Here's how the part is built. I have some questions about the finished solid (model axes, mm). A direction names the side the tool comes from. Round coordinates to 2 decimals unless told otherwise and drop trailing zeros. Loops run counter-clockwise (first coordinate to the right, second up) from the corner with the lowest first, then second, coordinate; pieces in that order, holes last. Notation, with made-up numbers: M 48.25,-24.5 L 77.25,-24.5 A11 ccw 77.25,-14.5 Z; hole C 77,25 d10. An arc over 180 degrees is marked long. Use a Markdown table: item, result.
```python
from build123d import *

# Parameters (mm, degrees)
BOSS_EXTRUDE1_DEPTH = 215.9


with BuildPart() as part:
    # Sketch1 → Boss-Extrude1 (new body)
    with BuildSketch(Plane(origin=(0, 0, 0), x_dir=(0, 0, -1), z_dir=(1, 0, 0))):
        with BuildLine():
            Line((0, 0), (30, 0))
            Line((30, 0), (30, 5))
            Line((30, 5), (27.221875, 7.778125))
            Line((27.221875, 7.778125), (27.221875, 14.278125))
            ThreePointArc((27.221875, 14.278125), (28.035568974, 16.242556026), (30, 17.05625))
            Line((30, 17.05625), (30, 20.221875))
            ThreePointArc((30, 20.221875), (28.035568974, 21.035568974), (27.221875, 23))
            Line((27.221875, 23), (2.778125, 23))
            ThreePointArc((2.778125, 23), (1.964431026, 21.035568974), (0, 20.221875))
            Line((0, 20.221875), (0, 17.05625))
            ThreePointArc((0, 17.05625), (1.964431026, 16.242556026), (2.778125, 14.278125))
            Line((2.778125, 14.278125), (2.778125, 7.778125))
            Line((2.778125, 7.778125), (0, 5))
            Line((0, 5), (0, 0))
        make_face()
    extrude(amount=BOSS_EXTRUDE1_DEPTH)


solid = part.part
```
Q1. Will these pins go through, and if not, where does the flat tip stop? P1, Ø1.9, axis at x = 133, y = 10, coming from the -Z side; P2, Ø3, axis at x = 63, y = 8.5, coming from the +Z side; P3, Ø3, axis at x = 93, y = 11, coming from the +Z side.
Return value:
| item | result |
|---|---|
| P1 | stops at z = -27.22 |
| P2 | stops at z = -2 |
| P3 | stops at z = -2.78 |
Q2. For faces 1 (the flat face through (106, 11, -2.778)), 2 (the flat face through (106, 11, -27.222)), 3 (the flat face through (106, 0, -15)), which set-ups out of +Z, -Z, +X, -X, +Y, -Y let a thin tool reach every point of the face, with its end or its side?
Return value:
| item | result |
|---|---|
| face 1 | +Z, +X, -X |
| face 2 | -Z, +X, -X |
| face 3 | +Z, -Z, +X, -X, -Y |
Q3. I need wall thicknesses on line 1 (Y direction, x = 188.5, z = -1.25); line 2 (Z direction, x = 116, y = 12); line 3 (Z direction, x = 202.5, y = 7.5). Which ranges of each line are inside material? Lowest first, please. Write a range as from..to.
Return value:
| item | result |
|---|---|
| line 1 | y = 0..6.25, 16.76..20.52 |
| line 2 | z = -27.22..-2.78 |
| line 3 | z = -27.5..-2.5 |
Q4. Imagine slicing it at A-A, the plane x = 67. Please give me the cut outline in (y, z).
Return value:
| item | result |
|---|---|
| outline | M 0,-30 L 5,-30 L 7.78,-27.22 L 14.28,-27.22 A2.78 cw 17.06,-30 L 20.22,-30 A2.78 cw 23,-27.22 L 23,-2.78 A2.78 cw 20.22,0 L 17.06,0 A2.78 cw 14.28,-2.78 L 7.78,-2.78 L 5,0 L 0,0 Z |
